Can you work these out from the model? Positions are in its coordinate system, mm. Face numbers are marked on the shaded views. A direction names the side the tool comes from. Give positions to 0.01 mm unless a question says otherwise; leave off trailing zeros. Order: outer loops, then holes, each group sorted by start corner. A loop starts at its lowest first (then second) coordinate and runs counter-clockwise, first axis right, second up. Notation, with made-up numbers: (64, -17) - (119, -17) arc R29 ccw to (119, 4) - close; hole circle Ø10 at (34.5, 37.5). An arc over 180 degrees is marked (long way). Answer as CSV lines item,"result".
```python
from build123d import *

# Parameters (mm, degrees)
F0_R     = 15.875
F1_DEPTH = 50.8
F2_R     = 12.827
F3_DEPTH = 38.1
F5_DEPTH = 12.7
F6_R     = 3.373438
F7_DEPTH = 15.875


with BuildPart() as f1:
    # F0 (on Front) → F1 (new body)
    with BuildSketch(Plane.XZ):
        Circle(F0_R)
    extrude(amount=F1_DEPTH)

    # F2 (on face) → F3 (cut)
    with BuildSketch(Plane.XZ.offset(50.8)):
        Circle(F2_R)
    extrude(amount=-F3_DEPTH, mode=Mode.SUBTRACT)

    # F4 (on face) → F5 (cut)
    with BuildSketch(Plane.XZ.offset(12.7)):
        Polygon((7.405636, -0.023035), (3.722767, 6.401951), (-3.682869, 6.424986), (-7.405636, 0.023035), (-3.722767, -6.401951), (3.682869, -6.424986), align=None)
    extrude(amount=-F5_DEPTH, mode=Mode.SUBTRACT)

    # F6 (on Right) → F7 (cut, symmetric)
    with BuildSketch(Plane.YZ):
        with Locations((-31.75, 0)):
            Circle(F6_R)
    extrude(amount=F7_DEPTH, both=True, mode=Mode.SUBTRACT)


solid = f1.part
```
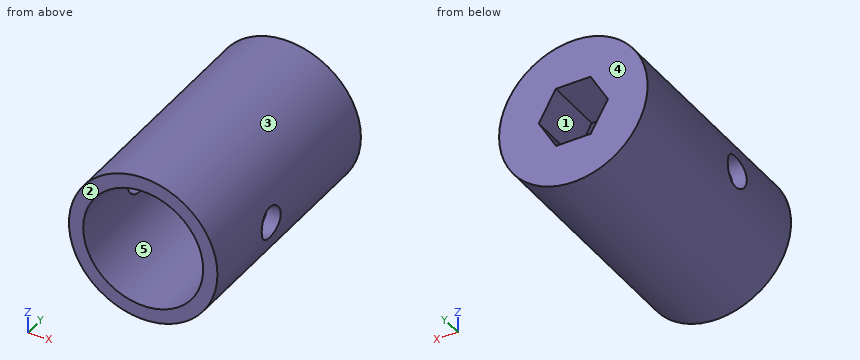
1) If we mould it in two halves opening along X, with no side actions, what happens to the marked faces 3, 4 and 5? For each: +X half, -X half, draft (parallel to the pull), parting line (faces both ways), or undercut.
Answer block:
face 3,"parting line"
face 4,"draft"
face 5,"undercut"
2) I want a section at C-C on y = -5.5. Write out the boundary of the cut face in (x, z) (3 decimals), plus the area to 3 significant figures.
Answer block:
outline,"circle Ø31.75 at (0, 0); hole (-7.406, 0.023) - (-3.723, -6.402) - (3.683, -6.425) - (7.406, -0.023) - (3.723, 6.402) - (-3.683, 6.425) - close"
area,"649 mm2"
3) I want a section at B-B on x = 0. Write out the boundary of the cut face in (y, z) (3 decimals).
Answer block:
outline,"(-50.8, -15.875) - (0, -15.875) - (0, -6.414) - (-12.7, -6.414) - (-12.7, -12.827) - (-50.8, -12.827) - close; (-50.8, 12.827) - (-12.7, 12.827) - (-12.7, 6.414) - (0, 6.414) - (0, 15.875) - (-50.8, 15.875) - close"
4) I want a section at D-D on z = -1. Write out the boundary of the cut face in (x, y), plus the area to 3 significant figures.
Answer block:
outline,"(-15.84, -50.8) - (-12.79, -50.8) - (-12.79, -34.97) - (-15.84, -34.97) - close; (-15.84, -28.53) - (-12.79, -28.53) - (-12.79, -12.7) - (-6.82, -12.7) - (-6.82, 0) - (-15.84, 0) - close; (6.84, -12.7) - (12.79, -12.7) - (12.79, -28.53) - (15.84, -28.53) - (15.84, 0) - (6.84, 0) - close; (12.79, -50.8) - (15.84, -50.8) - (15.84, -34.97) - (12.79, -34.97) - close"
area,"422 mm2"
5) I want a section at A-A on y = -32.5. Write out the boundary of the cut face in (x, z) (3 decimals), plus the area to 3 significant figures.
Answer block:
outline,"(-15.531, -3.289) arc R15.875 ccw to (15.531, -3.289) - (12.398, -3.289) arc R12.827 cw to (-12.398, -3.289) - close; (-15.531, 3.289) - (-12.398, 3.289) arc R12.827 cw to (12.398, 3.289) - (15.531, 3.289) arc R15.875 ccw to start"
area,"234 mm2"
6) Which directions (+Z, -Z, +X, -X, +Y, -Y) give clear straight access to the entire face, cutting with the end or side of a thin tool? Please do the marked faces 1 and 2.
Answer block:
face 1,"+Y, -Y"
face 2,"+Z, -Z, +X, -X, -Y"
7) I need wall thicknesses on line 1 along X through (y, z) = (-36, 0) (3 decimals); line 2 along Y through (x, z) = (-2.5, -11.5). Which ranges of each line are inside material? Lowest first, please. Write a range as [from, to].
Answer block:
line 1,"[-15.875, -12.827], [12.827, 15.875]"
line 2,"[-12.7, 0]"
8) I'm going to push flat-ended pins straight in: P1, Ø1.5, axis at x = -2, y = -33.5, coming from the +Z side; P2, Ø2, axis at y = -40.5, z = -12.5, coming from the -X side; P3, Ø1, axis at y = -38.5, z = -6.5, coming from the +X side; P4, Ø4, axis at y = -31.75, z = 0, coming from the -X side. Where does each tip first touch, or does it pass through?
Answer block:
P1,"z = 15.83"
P2,"x = -10.94"
P3,"x = 14.7"
P4,"through"
